Design review of the part built by this model. Coordinates are the model's own, in mm. Face numbers are marked on the shaded views. A direction names the side the tool comes from. Round coordinates to 2 decimals unless told otherwise and drop trailing zeros. Write each loop counter-clockwise with the first axis right and the second up, starting at its lowest first coordinate (ties: lowest second). Pieces come first, ordered by that corner, then holes. Notation, with made-up numbers: (53, 26.5) -> (76, 26.5) arc R31 cw to (76, 53.5) -> close; hole circle Ø3 at (-31.75, 27.25). An arc over 180 degrees is marked (long way). Write item = value, one per line. Start each with the question number.
Item 1: Add section B-B, the plane x = -25. State the section outline as (y, z) points, then the cut area to 3 significant figures.
Item 2: Add section A-A, the plane y = 16. State how many separate pieces and enclosed holes the cut face has, then the cut area to 3 significant figures.
Item 3: For pin 1 Ø1.9 at (x, z) = (0.5, -24) entering from +Y; pin 2 Ø1.8 at (x, z) = (-25, -25) entering from -Y, all flat-tipped, find the tip position at first contact; note any pin that passes through.
Item 4: Add section C-C, the plane z = -25. State the section outline as (x, y) points.
Item 5: Mouldability with a two-part tool opening along Z and no side actions: class the marked faces 3, 4 and 5 as released by +Z, released by -Z, zero draft, split by the parting line, or undercut.
Item 6: Add section D-D, the plane x = 0. State the section outline as (y, z) points, then the cut area to 3 significant figures.
Item 7: To check wall thickness, follow L1, parallel to X at y = 18, z = -25; L2, parallel to Z at x = 25, y = 4. State the ranges of each line that lie inside material, in increasing order.
Item 8: Machinability: for the marked faces 1 and 2, which of the approach directions +Z, -Z, +X, -X, +Y, -Y give a long, thin tool a straight path to every point of the face, cutting with its end or side? Answer none if there is none.
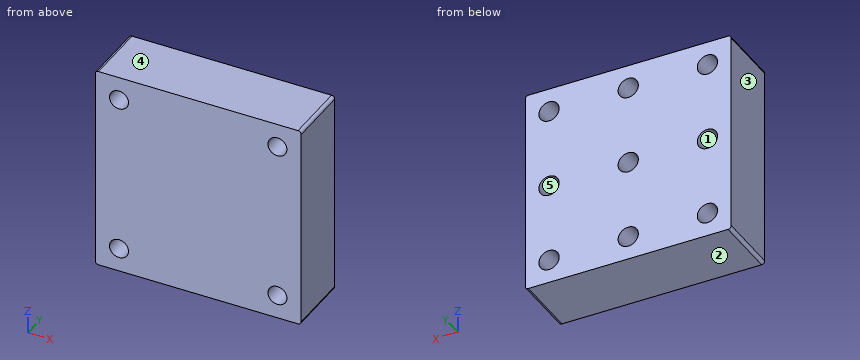
from build123d import *

# Parameters (mm, degrees)
SKETCH_1_W          = 65
SKETCH_1_H          = 65
EXTRUDE_1_DEPTH     = 20
SKETCH_2_R          = 3
CUT_EXTRUDE_1_DEPTH = 7.5
SKETCH_3_R          = 3.2
CUT_EXTRUDE_2_DEPTH = 7.5
FILLET_1_R          = 1


with BuildPart() as part:
    # 스케치1 → 보스-돌출1 (new body)
    with BuildSketch(Plane(origin=(0, 0, 0), x_dir=(1, 0, 0), z_dir=(0, 1, 0))):
        Rectangle(SKETCH_1_W, SKETCH_1_H)
    extrude(amount=EXTRUDE_1_DEPTH)

    # 스케치2 → 컷-돌출1 (cut)
    with BuildSketch(Plane.XZ):
        with Locations((-25, 25)):
            Circle(SKETCH_2_R)
        with Locations((25, 25)):
            Circle(SKETCH_2_R)
        with Locations((25, -25)):
            Circle(SKETCH_2_R)
        with Locations((-25, -25)):
            Circle(SKETCH_2_R)
    extrude(amount=-CUT_EXTRUDE_1_DEPTH, mode=Mode.SUBTRACT)

    # 스케치3 → 컷-돌출2 (cut)
    with BuildSketch(Plane(origin=(0, 20, 0), x_dir=(1, 0, 0), z_dir=(0, 1, 0))):
        with Locations((-25, 25)):
            Circle(SKETCH_3_R)
        with Locations((0, 25)):
            Circle(SKETCH_3_R)
        with Locations((25, 25)):
            Circle(SKETCH_3_R)
        with Locations((25, 0)):
            Circle(SKETCH_3_R)
        with Locations((25, -25)):
            Circle(SKETCH_3_R)
        with Locations((0, -25)):
            Circle(SKETCH_3_R)
        with Locations((-25, -25)):
            Circle(SKETCH_3_R)
        with Locations((-25, 0)):
            Circle(SKETCH_3_R)
        Circle(SKETCH_3_R)
    extrude(amount=-CUT_EXTRUDE_2_DEPTH, mode=Mode.SUBTRACT)

    # 필렛1
    fillet_1_edges = [part.edges().sort_by_distance(p)[0] for p in [
        (-32.5, 10, -32.5),
        (32.5, 10, -32.5),
        (32.5, 10, 32.5),
        (-32.5, 10, 32.5),
    ]]
    fillet(fillet_1_edges, radius=FILLET_1_R)


solid = part.part
Result set:
q1.outline = (0, -32.5) -> (20, -32.5) -> (20, -28.2) -> (12.5, -28.2) -> (12.5, -21.8) -> (20, -21.8) -> (20, -3.2) -> (12.5, -3.2) -> (12.5, 3.2) -> (20, 3.2) -> (20, 21.8) -> (12.5, 21.8) -> (12.5, 28.2) -> (20, 28.2) -> (20, 32.5) -> (0, 32.5) -> (0, 28) -> (7.5, 28) -> (7.5, 22) -> (0, 22) -> (0, -22) -> (7.5, -22) -> (7.5, -28) -> (0, -28) -> close
q1.area = 1,070 mm²
q2.separate_pieces = 1
q2.enclosed_holes = 9
q2.area = 3,930 mm²
q3.pin_1 = 12.5
q3.pin_2 = 7.5
q4.outline = (-32.5, 0) -> (-28, 0) -> (-28, 7.5) -> (-22, 7.5) -> (-22, 0) -> (22, 0) -> (22, 7.5) -> (28, 7.5) -> (28, 0) -> (32.5, 0) -> (32.5, 20) -> (28.2, 20) -> (28.2, 12.5) -> (21.8, 12.5) -> (21.8, 20) -> (3.2, 20) -> (3.2, 12.5) -> (-3.2, 12.5) -> (-3.2, 20) -> (-21.8, 20) -> (-21.8, 12.5) -> (-28.2, 12.5) -> (-28.2, 20) -> (-32.5, 20) -> close
q5.face_3 = zero draft
q5.face_4 = released by +Z
q5.face_5 = undercut
q6.outline = (0, -32.5) -> (20, -32.5) -> (20, -28.2) -> (12.5, -28.2) -> (12.5, -21.8) -> (20, -21.8) -> (20, -3.2) -> (12.5, -3.2) -> (12.5, 3.2) -> (20, 3.2) -> (20, 21.8) -> (12.5, 21.8) -> (12.5, 28.2) -> (20, 28.2) -> (20, 32.5) -> (0, 32.5) -> close
q6.area = 1,160 mm²
q7.L1 = -32.5 to -28.2, -21.8 to -3.2, 3.2 to 21.8, 28.2 to 32.5
q7.L2 = -32.5 to -28, -22 to 22, 28 to 32.5
q8.face_1 = +Y
q8.face_2 = -Z, +X, -X, +Y, -Y
